Could you check a few things on this model? Use its own coordinates, in mm. A direction names the side the tool comes from. Coordinates: 2 decimals unless noted, no trailing zeros. Write each loop counter-clockwise with the first axis right and the second up, starting at its lowest first coordinate (ties: lowest second). Pieces come first, ordered by that corner, then holes.
```python
from build123d import *

# Parameters (mm, degrees)
SKETCH_1_R      = 31.5
EXTRUDE_1_DEPTH = 16
SKETCH_2_R      = 32.5
SKETCH_2_R_2    = 31.5
EXTRUDE_2_DEPTH = 11
CHAMFER_1_SIZE  = 1


with BuildPart() as part:
    # 草图1 → 凸台-拉伸1 (new, symmetric)
    with BuildSketch(Plane(origin=(0, 0, 0), x_dir=(1, 0, 0), z_dir=(0, 1, 0))):
        with Locations(Location((0, 0, 0), (0, 0, 270))):
            Circle(SKETCH_1_R)
        with BuildLine():
            Line((-3, 9.539392014), (-3, 11.7))
            Line((-3, 11.7), (3, 11.7))
            Line((3, 11.7), (3, 9.539392014))
            ThreePointArc((3, 9.539392014), (0, -10), (-3, 9.539392014))
        make_face(mode=Mode.SUBTRACT)
    extrude(amount=EXTRUDE_1_DEPTH, both=True)

    # 草图2 → 凸台-拉伸2 (add, symmetric)
    with BuildSketch(Plane(origin=(0, 0, 0), x_dir=(1, 0, 0), z_dir=(0, 1, 0))):
        with Locations(Location((0, 0, 0), (0, 0, 270))):
            Circle(SKETCH_2_R)
        with Locations(Location((0, 0, 0), (0, 0, 270))):
            Circle(SKETCH_2_R_2, mode=Mode.SUBTRACT)
    extrude(amount=EXTRUDE_2_DEPTH, both=True)

    # 倒角1
    chamfer_1_edges = [part.edges().sort_by_distance(p)[0] for p in [
        (0, -16, -31.5),
        (0, 16, -31.5),
    ]]
    chamfer(chamfer_1_edges, length=CHAMFER_1_SIZE)


solid = part.part
```
1. I want a section at A-A on x = 0. Please give me the cut outline in (y, z), plus the area to 3 significant figures.
Verdict:
outline: (-16, -30.5) - (-15, -31.5) - (-11, -31.5) - (-11, -32.5) - (11, -32.5) - (11, -31.5) - (15, -31.5) - (16, -30.5) - (16, -11.7) - (-16, -11.7) - close; (-16, 10) - (16, 10) - (16, 30.5) - (15, 31.5) - (11, 31.5) - (11, 32.5) - (-11, 32.5) - (-11, 31.5) - (-15, 31.5) - (-16, 30.5) - close
area: 1,360 mm2
2. I want a section at D-D on y = 3.5. Please give me the cut outline in (x, z), plus the area to 3 significant figures.
Verdict:
outline: circle Ø65 at (0, 0); hole (-3, -11.7) - (3, -11.7) - (3, -9.54) arc R10 ccw (long way) to (-3, -9.54) - close
area: 2,990 mm2
3. Please list where these lines run through material, in increasing order: line 1 along X through (y, z) = (7, 0); line 2 along Z through (x, y) = (-6, -10); line 3 along Z through (x, y) = (-4.5, 8).
Verdict:
line 1: x = -32.5 to -10, 10 to 32.5
line 2: z = -31.94 to -8, 8 to 31.94
line 3: z = -32.19 to -8.93, 8.93 to 32.19
4. If we mould it in two halves opening along X, with no side actions, what happens to faces 1 (the face through (9.76, 0.15, 31)), 2 (the face through (0, 0, -11.7)), 3 (the face through (7.2, -16, -7.2))? For each: pulls with the +X half, pulls with the -X half, needs draft (parallel to the pull), parting line crosses it, or undercut.
Verdict:
face 1: parting line crosses it
face 2: undercut
face 3: needs draft
5. On a 3-axis mill with a long thin cutter (end or side, diameter ignored), from which of +Z, -Z, +X, -X, +Y, -Y can I reach the whole of each face in a straight line? I mean faces 4 (the face through (7.2, 16, -7.2)), 5 (the face through (27, 11, -17)), 6 (the face through (31.232, -12.972, -4.101)), 7 (the face through (-3, 0, -11)). Say none if no direction works.
Verdict:
face 4: +Z, -Z, +X, -X, +Y
face 5: +Y
face 6: -Y
face 7: +Y, -Y
6. I want a section at C-C on y = 12.5. Please give me the cut outline in (x, z), plus the area to 3 significant figures.
Verdict:
outline: circle Ø63 at (0, 0); hole (-3, -11.7) - (3, -11.7) - (3, -9.54) arc R10 ccw (long way) to (-3, -9.54) - close
area: 2,790 mm2
7. I want a section at B-B on z = 0. Please give me the cut outline in (x, y).
Verdict:
outline: (-32.5, -11) - (-31.5, -11) - (-31.5, -15) - (-30.5, -16) - (-10, -16) - (-10, 16) - (-30.5, 16) - (-31.5, 15) - (-31.5, 11) - (-32.5, 11) - close; (10, -16) - (30.5, -16) - (31.5, -15) - (31.5, -11) - (32.5, -11) - (32.5, 11) - (31.5, 11) - (31.5, 15) - (30.5, 16) - (10, 16) - close
8. For pin 1 (1.7 mm diameter, centred on y = 6, z = -10.5, fed in from +X); pin 2 (1.5 mm diameter, centred on x = -12, y = 6.5, fed in from +Z); pin 3 (4 mm diameter, centred on y = -10.5, z = -2.5, fed in from -X), each with a flat end and sliding along its axis, tell me the tip position at first contact or that it passes through.
Verdict:
pin 1: stops at x = 31.03
pin 2: stops at z = 30.49
pin 3: stops at x = -32.5
